Verification items for the finished model (mm, model axes). Round coordinates to 2 decimals unless told otherwise and drop trailing zeros. Order: outer loops, then holes, each group sorted by start corner. A loop starts at its lowest first (then second) coordinate and runs counter-clockwise, first axis right, second up. Notation, with made-up numbers: (10.5, 45.25) -> (61.5, 45.25) arc R11 ccw to (61.5, 61.25) -> close; hole circle Ø7 at (-14, 85). An arc over 180 degrees is marked (long way). Answer in a Markdown table with one row per item. Add a question column.
```python
from build123d import *

# Parameters (mm, degrees)
SKETCH1_W           = 98.044
SKETCH1_H           = 25.4
BOSS_EXTRUDE1_DEPTH = 29.21
FILLET1_R           = 12
FILLET2_R           = 1


with BuildPart() as part:
    # Sketch1 → Boss-Extrude1 (new body)
    with BuildSketch(Plane(origin=(0, 0, 0), x_dir=(1, 0, 0), z_dir=(0, 1, 0))):
        Rectangle(SKETCH1_W, SKETCH1_H)
    extrude(amount=BOSS_EXTRUDE1_DEPTH)

    # Fillet1
    fillet1_edges = [part.edges().sort_by_distance(p)[0] for p in [
        (49.022, 14.605, 12.7),
        (49.022, 14.605, -12.7),
    ]]
    fillet(fillet1_edges, radius=FILLET1_R)

    # Fillet2
    fillet2_edges = [part.edges().sort_by_distance(p)[0] for p in [
        (-49.022, 14.605, 12.7),
        (-49.022, 14.605, -12.7),
    ]]
    fillet(fillet2_edges, radius=FILLET2_R)


solid = part.part
```
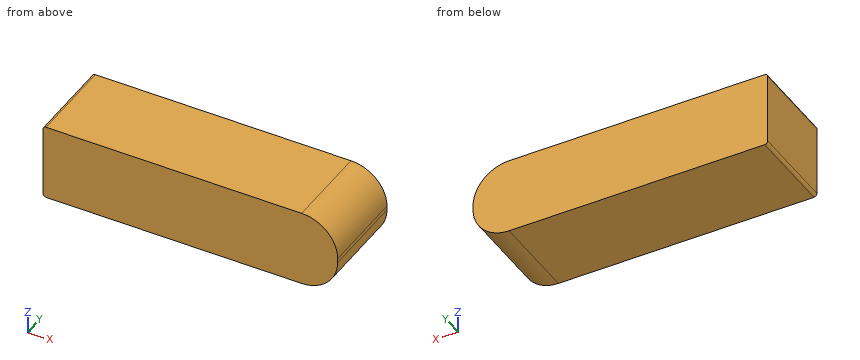
1) Thickness scan on L1, parallel to X at y = 17, z = 3.5; L2, parallel to X at y = 2, z = -5. Record the ranges inside material, lowest first. Write a range as [from, to].
2) Cross-section at C-C, the plane z = 8.5. Record the boundary of the cut face in (x, y), and give its area (3 significant figures).
3) Cross-section at A-A, the plane y = 22.5. Record the boundary of the cut face in (x, z).
4) Cross-section at B-B, the plane z = -6.75. Record the boundary of the cut face in (x, y).
5) Depth check by flat-ended pin: P1, Ø1.5, axis at y = 7, z = 3, coming from the +X side; P2, Ø1, axis at x = 39, y = 15.5, coming from the -Z side; P3, Ø5, axis at y = 7.5, z = -6, coming from the +X side. Enter the tip coordinate at first touch or a pass-through.
Results below:
| question | item | result |
|---|---|---|
| 1 | L1 | [-49.02, 48.69] |
| 1 | L2 | [-49.02, 48.23] |
| 2 | outline | (-49.02, 0) -> (46.14, 0) -> (46.14, 29.21) -> (-49.02, 29.21) -> close |
| 2 | area | 2,780 mm² |
| 3 | outline | (-49.02, -11.7) arc R1 ccw to (-48.02, -12.7) -> (37.02, -12.7) arc R12 ccw to (49.02, -0.7) -> (49.02, 0.7) arc R12 ccw to (37.02, 12.7) -> (-48.02, 12.7) arc R1 ccw to (-49.02, 11.7) -> close |
| 4 | outline | (-49.02, 0) -> (47.39, 0) -> (47.39, 29.21) -> (-49.02, 29.21) -> close |
| 5 | P1 | x = 48.92 |
| 5 | P2 | z = -12.61 |
| 5 | P3 | x = 48.69 |
